The model under review builds one solid part; all positions refer to its coordinate system, in mm. A direction names the side the tool comes from. Round coordinates to 2 decimals unless told otherwise and drop trailing zeros. Order: outer loops, then holes, each group sorted by start corner. A loop starts at its lowest first (then second) coordinate and runs counter-clockwise, first axis right, second up. Notation, with made-up numbers: M -20,12 L 12,12 A20 cw 12,34 Z; hole C 8,-16.5 d2. An arc over 180 degrees is marked long. Answer as a JSON object with one key per item and string values. Group by question number.
1) Consider section C-C, the plane x = -12.5. Write out the cut boundary in (y, z) (3 decimals).
2) The part is to be moulded in two halves that separate along Y. For faces 1 (the flat face through (-17.78, 18, -110)), 2 (the flat face through (-19.05, 18, -110)), 3 (the flat face through (-3, 0, -110)), say which applies: +Y half, -Y half, draft (parallel to the pull), parting line (faces both ways), or undercut.
3) Consider section A-A, the plane x = -2.5. Write out the cut boundary in (y, z) (3 decimals), then the cut area to 3 significant figures.
4) To check wall thickness, follow line 1 (Y direction, x = -1, z = -121.5) (3 decimals); line 2 (X direction, y = 19, z = -145.5); line 3 (X direction, y = 21.25, z = -17.5). State the ranges of each line that lie inside material, in increasing order.
5) For faces 4 (the flat face through (-3, 1.27, -110)), 5 (the cylindrical face through (-9.914, 9.53, -109.569)), list the 3-axis set-ups (+Z, -Z, +X, -X, +Y, -Y) from which the entire face can be reached by the end or side of a thin tool; tool diameter is ignored.
6) Insertion check: pin 1 Ø1 at (y, z) = (17.5, -127.5) entering from +X; pin 2 Ø1 at (y, z) = (3, -98.5) entering from -X; pin 3 Ø6 at (y, z) = (17.5, -68.5) entering from +X. Each pin has a flat end and moves straight along its axis. Give the tip position at first contact, or say it passes through.
7) Consider section D-D, the plane y = 9.5. Write out the cut boundary in (x, z).
```python
from build123d import *

# Parameters (mm, degrees)
EXTRUDE_THIN1_DEPTH = 222.25
FILLET1_R           = 1.27


with BuildPart() as part:
    # Sketch1 → Extrude-Thin1 (new body)
    with BuildSketch(Plane.XY):
        with BuildLine():
            Line((0, 0), (-6.35, 0))
            ThreePointArc((-6.35, 0), (-9.958615648, 9.580536091), (-19.05, 14.2875))
            Line((-19.05, 14.2875), (-19.05, 22.225))
            Line((-19.05, 22.225), (0, 22.225))
            Line((0, 22.225), (0, 20.955))
            Line((0, 20.955), (-17.78, 20.955))
            Line((-17.78, 20.955), (-17.78, 15.381314))
            ThreePointArc((-17.78, 15.381314), (-9.055144579, 10.475506123), (-5.12465987, 1.27))
            Line((-5.12465987, 1.27), (0, 1.27))
            Line((0, 1.27), (0, 0))
        make_face()
    extrude(amount=-EXTRUDE_THIN1_DEPTH)

    # Fillet1
    fillet1_edges = [part.edges().sort_by_distance(p)[0] for p in [
        (-6.35, 0, -111.125),
        (-19.05, 14.2875, -111.125),
        (-19.05, 22.225, -111.125),
    ]]
    fillet(fillet1_edges, radius=FILLET1_R)


solid = part.part
```
Results list:
{
 "1": {"outline": "M 11.832,-222.25 L 13.348,-222.25 L 13.348,0 L 11.832,0 Z; M 20.955,-222.25 L 22.225,-222.25 L 22.225,0 L 20.955,0 Z"},
 "2": {"face 1": "undercut", "face 2": "draft", "face 3": "-Y half"},
 "3": {"outline": "M 0,-222.25 L 1.27,-222.25 L 1.27,0 L 0,0 Z; M 20.955,-222.25 L 22.225,-222.25 L 22.225,0 L 20.955,0 Z", "area": "565 mm^2"},
 "4": {"line 1": "0 to 1.27, 20.955 to 22.225", "line 2": "-19.05 to -17.78", "line 3": "-19.02 to 0"},
 "5": {"face 4": "+Z, -Z, +X", "face 5": "+Z, -Z, -X, -Y"},
 "6": {"pin 1": "x = -17.78", "pin 2": "x = -6.76", "pin 3": "x = -14.78"},
 "7": {"outline": "M -9.89,-222.25 L -8.25,-222.25 L -8.25,0 L -9.89,0 Z"}
}
